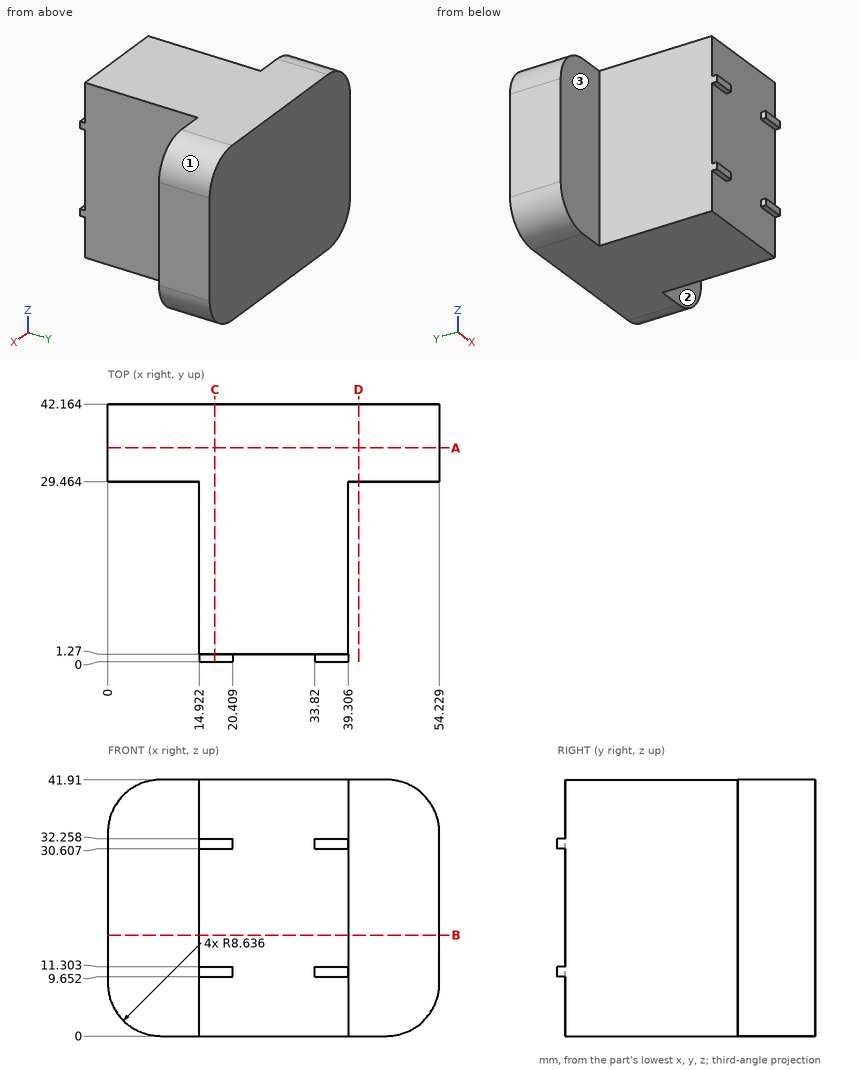
Answer from the drawing. Dimensions are ordinates in mm from the lowest x, y and z of the part. A direction names the side the tool comes from. Round coordinates to 2 decimals unless told otherwise and drop trailing zeros. Loops run counter-clockwise (first coordinate to the right, second up) from the corner with the lowest first, then second, coordinate; pieces in that order, holes last. Notation, with made-up numbers: (9.5, 9.25) - (51.5, 9.25) arc R15 ccw to (51.5, 31.25) - close; hole circle Ø8 at (-8, 82). An arc over 180 degrees is marked (long way). Return JSON: item names as keys, results as strings. Group by question number.
1. Consider probe 1 along X at (y, z) = (5.5, 3); probe 2 along Y at (x, z) = (39, 16) (1 decimal); probe 3 along Y at (x, z) = (14.5, 4) (1 decimal). Determine where each line is inside the solid, lowest interval first.
2. Which of the six approach directions +Z, -Z, +X, -X, +Y, -Y give full straight-line access (tool end or side, diameter ignored) to the marked faces 1, 2 and 3?
3. The part is cut by section D-D on x = 41. Determine the outline of the cut face in (y, z) (1 decimal).
4. The part is cut by section C-C on x = 17.5. Determine the outline of the cut face in (y, z) (1 decimal), then the cut area to 3 significant figures.
5. Each of these flat-tipped pins is pushed along its axis until it touches: P1, Ø7.5, axis at x = 28.5, z = 26.5, coming from the -Y side; P2, Ø1, axis at y = 1, z = 10.5, coming from the +X side; P3, Ø10, axis at x = 6, z = 28, coming from the -Y side; P4, Ø1, axis at x = 27, y = 24, coming from the -Z side. Where does it stop, or does it pass through?
6. The part is cut by section B-B on z = 16.5. Determine the outline of the cut face in (x, y) (1 decimal), then the cut area to 3 significant figures.
7. The part is cut by section A-A on y = 35. Determine the outline of the cut face in (x, z) (1 decimal).
Resolved:
{
 "1": {"probe 1": "x = 14.92 to 39.31", "probe 2": "y = 1.3 to 42.2", "probe 3": "y = 29.5 to 42.2"},
 "2": {"face 1": "+Z, +X, +Y, -Y", "face 2": "+Z, -Z, +X, -Y", "face 3": "+Z, -Z, -X, -Y"},
 "3": {"outline": "(29.5, 0) - (42.2, 0) - (42.2, 41.9) - (29.5, 41.9) - close"},
 "4": {"outline": "(0, 9.7) - (1.3, 9.7) - (1.3, 0) - (42.2, 0) - (42.2, 41.9) - (1.3, 41.9) - (1.3, 32.3) - (0, 32.3) - (0, 30.6) - (1.3, 30.6) - (1.3, 11.3) - (0, 11.3) - close", "area": "1,720 mm²"},
 "5": {"P1": "stops at y = 1.27", "P2": "stops at x = 39.31", "P3": "stops at y = 29.46", "P4": "stops at z = 0"},
 "6": {"outline": "(0, 29.5) - (14.9, 29.5) - (14.9, 1.3) - (39.3, 1.3) - (39.3, 29.5) - (54.2, 29.5) - (54.2, 42.2) - (0, 42.2) - close", "area": "1,380 mm²"},
 "7": {"outline": "(0, 8.6) arc R8.6 ccw to (8.6, 0) - (45.6, 0) arc R8.6 ccw to (54.2, 8.6) - (54.2, 33.3) arc R8.6 ccw to (45.6, 41.9) - (8.6, 41.9) arc R8.6 ccw to (0, 33.3) - close"}
}
